from build123d import *
from build123d.topology import SkipClean

# Parameters (mm, degrees)
SKETCH1_R           = 20
SKETCH1_R_2         = 10
BOSS_EXTRUDE1_DEPTH = 7
SKETCH2_R           = 30
SKETCH2_R_2         = 10
BOSS_EXTRUDE2_DEPTH = 2
SKETCH3_R           = 2
CUT_EXTRUDE1_DEPTH  = 45.09081537
CUT_EXTRUDE2_DEPTH  = 46.343136195


with BuildPart() as part:
    # Sketch1 → Boss-Extrude1 (new, symmetric)
    with BuildSketch(Plane(origin=(0, 0, 0), x_dir=(0, 0, -1), z_dir=(1, 0, 0))):
        Circle(SKETCH1_R)
        Circle(SKETCH1_R_2, mode=Mode.SUBTRACT)
    extrude(amount=BOSS_EXTRUDE1_DEPTH, both=True)

    # Sketch2 → Boss-Extrude2 (add, symmetric)
    with BuildSketch(Plane.ZY.offset(7)):
        Circle(SKETCH2_R)
        Circle(SKETCH2_R_2, mode=Mode.SUBTRACT)
    extrude(amount=BOSS_EXTRUDE2_DEPTH, both=True)

    # Sketch3 → Cut-Extrude1 (cut, through all)
    with BuildSketch(Plane(origin=(-5, 0, 0), x_dir=(0, 0, -1), z_dir=(1, 0, 0))):
        with Locations((0, 25)):
            Circle(SKETCH3_R)
        with Locations((25, 0)):
            Circle(SKETCH3_R)
        with Locations((0, -25)):
            Circle(SKETCH3_R)
        with Locations((-25, 0)):
            Circle(SKETCH3_R)
    extrude(amount=-CUT_EXTRUDE1_DEPTH, mode=Mode.SUBTRACT)

    # Sketch4 → Cut-Extrude2 (cut, through all)
    with SkipClean():  # the faces are left unmerged after this step: merging them gives an invalid solid
        with BuildSketch(Plane(origin=(7, 0, 0), x_dir=(0, 0, -1), z_dir=(1, 0, 0))):
            with BuildLine():
                ThreePointArc((-2, 9.797958971), (-1.00508962, 9.94936153), (0, 10))
                Line((0, 10), (0, 10.797958971))
                Line((0, 10.797958971), (-2, 10.797958971))
                Line((-2, 10.797958971), (-2, 9.797958971))
            make_face()
            with BuildLine():
                Line((0, 10.797958971), (0, 10))
                ThreePointArc((0, 10), (1.00508962, 9.94936153), (2, 9.797958971))
                Line((2, 9.797958971), (2, 10.797958971))
                Line((2, 10.797958971), (0, 10.797958971))
            make_face()
        extrude(amount=-CUT_EXTRUDE2_DEPTH, mode=Mode.SUBTRACT)


solid = part.part
Here's how the part is built. I have some questions about the finished solid (model axes, mm). Round coordinates to 2 decimals unless told otherwise and drop trailing zeros. Order: outer loops, then holes, each group sorted by start corner. A loop starts at its lowest first (then second) coordinate and runs counter-clockwise, first axis right, second up. Notation, with made-up numbers: M 58,8 L 62,8 A23 ccw 62,37 Z; hole C 88,88.5 d6. An arc over 180 degrees is marked long. Return JSON: item names as keys, results as strings. Group by question number.
1. If we section it at C-C on y = -25: List the corners of the cut face in (x, z) for me, then the cut area to 3 significant figures.
2. If we section it at A-A on z = -26: List the corners of the cut face in (x, y) for me.
3. Please list where these lines run through material, in increasing order: probe 1 along Y at (x, z) = (-5.75, 0); probe 2 along Y at (x, z) = (-1.5, 0); probe 3 along X at (y, z) = (26, 4.5).
4. If we section it at B-B on x = -7.75: List the corners of the cut face in (y, z) for me, then the cut area to 3 significant figures.
5. I'm going to push flat-ended pins straight in: pin 1 Ø5 at (x, y) = (-1.5, -11) entering from -Z; pin 2 Ø2 at (x, y) = (0.5, 5) entering from -Z; pin 3 Ø5 at (x, z) = (-2, 6.5) entering from -Y. Where does each tip first touch, or does it pass through?
6. If we mould it in two halves opening along Z, with no side actions, what happens to faces 1 (the face through (-5, 20.4, -0.4)), 2 (the face through (1.084, -19.524, 4.336)), 3 (the face through (-7, 0, -23))? For each: pulls with the +Z half, pulls with the -Z half, needs draft (parallel to the pull), parting line crosses it, or undercut.
7. If we section it at D-D on x = 4.25: List the corners of the cut face in (y, z) for me.
Reply:
{
 "1": {"outline": "M -9,-16.58 L -5,-16.58 L -5,-2 L -9,-2 Z; M -9,2 L -5,2 L -5,16.58 L -9,16.58 Z", "area": "117 mm^2"},
 "2": {"outline": "M -9,-14.97 L -5,-14.97 L -5,-1.73 L -9,-1.73 Z; M -9,1.73 L -5,1.73 L -5,14.97 L -9,14.97 Z"},
 "3": {"probe 1": "-30 to -27, -23 to -10, 10.8 to 23, 27 to 30", "probe 2": "-20 to -10, 10.8 to 20", "probe 3": "-9 to -5"},
 "4": {"outline": "C 0,0 d60; hole C -25,0 d4; hole C 0,-25 d4; hole C 0,25 d4; hole M 9.8,-2 L 10.8,-2 L 10.8,2 L 9.8,2 A10 ccw long Z; hole C 25,0 d4", "area": "2,460 mm^2"},
 "5": {"pin 1": "z = -18.1", "pin 2": "z = -19.6", "pin 3": "y = -19.6"},
 "6": {"face 1": "needs draft", "face 2": "parting line crosses it", "face 3": "undercut"},
 "7": {"outline": "C 0,0 d40; hole M 9.8,-2 L 10.8,-2 L 10.8,2 L 9.8,2 A10 ccw long Z"}
}
